Autodesk Inventor part; units mm, degrees
ref_plane "Work Plane1" through (6, 0, 0) normal (0, 0.5, 0.866) x (1, 0, 0)
ref_plane "YZ Plane" through (0, 0, 0) normal (1, 0, 0) x (0, 1, 0)
ref_plane "XZ Plane" through (0, 0, 0) normal (0, 1, 0) x (-1, 0, 0)
sketch "Sketch1" plane through (0, 0, 0) normal (0, 0, 1) x (1, 0, 0)
  line L0 (0, 0) -> (9.7226, 0)
  line L1 (12, 1.866) -> (12, 2.5)
  line L2 (12, 2.5) -> (0, 2.5)
  line L3 (12, 1.866) -> (10.8, 1.866)
  line L4 (10.8, 1.866) -> (9.7226, 0)
  line L5 (0, -0.5) -> (0, 3)
  line L6 (0, 2.5) -> (0, 0)
  dimension "d0" = 1.2
  dimension "d1" = 60
  dimension "d2" = 5
  dimension "d3" = 3.7321
  dimension "d5" = 12
revolve "Body" add sketch "Sketch1" angle 360 about axis through (0, 0, 0) along (1, 0, 0)
chamfer "Chamfer1" distance 0.3067 angle 60 1 edges at (12, -2.5, 0) measured on face at (12, 2.2645, -0.1994)
sketch "Sketch2" plane through (12, 0, 0) normal (1, 0, 0) x (0, 0, -1)
  circle A0 centre (0, 0) radius 1.866
  line L0 (-0.933, 1.616) -> (0.933, 1.616)
  line L1 (0.933, 1.616) -> (1.866, 0)
  line L2 (1.866, 0) -> (0.933, -1.616)
  line L3 (0.933, -1.616) -> (-0.933, -1.616)
  line L4 (-0.933, -1.616) -> (-1.866, 0)
  line L5 (-1.866, 0) -> (-0.933, 1.616)
  point P0 (0, 0)
  point P1 (0, 0)
extrude "Slot" add sketch "Sketch2" against normal up to next contours L1 A0 | A0 L2 | L0 A0 | A0 L3 | L5 A0 | A0 L4
thread "Thread"
chamfer "Chamfer2" distance 0.3067 angle 60 1 edges at (0, -2.5, 0) measured on face at (3.8229, 2.4919, -0.2012)
ref_plane "Work Plane1" through (6, 0, 0) normal (0, 0.5, 0.866) x (1, 0, 0)
equation "\"d0\" = INTI"
equation "\"d7\" = -0.5 * GD1 + 0.5 * NND"
equation "\"d8\" = FAWI"
equation "\"d29\" = -0.5 * GD1 + 0.5 * NND"
equation "\"d13\" = -0.5 * GD1 + 0.5 * NND"
equation "\"d14\" = FAWI"
equation "\"d30\" = -0.5 * GD1 + 0.5 * NND"
equation "\"NND\" = 3"
equation "\"NLG\" = 3"
equation "\"INTI\" = 1.2"
equation "\"FAWI\" = 60deg"
equation "\"SW\" = 1.5"
equation "\"GD1\" = THREADDIA - 1.2269 * PTC"
equation "\"FAWI1\" = 45deg"
equation "\"GUL\" = 0.61345 * PTC"
equation "\"SPD\" = 2"
equation "\"SEWI\" = 120deg"
equation "\"TOA\" = 30deg"
equation "\"THREADDIA\" = 3"
equation "\"PTC\" = 0.5"
equation "\"GAL\" = 0.61345 * PTC"
equation "\"E0\" = 1.155 * SW"
properties part number "Grub Screw 5x12mm" material "Stainless Steel, 440C"
Here's how the part is built. I have some questions about the finished solid (model axes, mm). A direction names the side the tool comes from. Coordinates: 2 decimals unless noted, no trailing zeros. Order: outer loops, then holes, each group sorted by start corner. A loop starts at its lowest first (then second) coordinate and runs counter-clockwise, first axis right, second up.
1) We'd pull the mould along Z, two halves only. Please class faces 3 (the face through (0, 0, 0)), 4 (the face through (5.81, -0.54, 2.44)), 5 (the face through (11.337, 0.819, -1.393)): +Z half, -Z half, draft (parallel to the pull), parting line (faces both ways), or undercut.
2) Will these pins go through, and if not, where does the flat tip stop? pin 1 (2 mm diameter, centred on x = 4, z = 2, fed in from +Y); pin 2 (1 mm diameter, centred on x = 9.5, y = 1.5, fed in from -Z).
3) Which directions (+Z, -Z, +X, -X, +Y, -Y) give clear straight access to the entire face, cutting with the end or side of a thin tool? Please do faces 1 (the face through (11.337, -0.797, -1.406)), 2 (the face through (12, -2, 0)).
4) I need wall thicknesses on line 1 (Y direction, x = 11, z = -0.55); line 2 (Y direction, x = 10.75, z = -0.35); line 3 (Y direction, x = 4.5, z = 1.2). Which ranges of each line are inside material? Lowest first, please.
5) Imagine slicing it at A-A on x = 1.5. List the corners of the cut face in (y, z) for me.
Response values:
1. face 3: draft
1. face 4: parting line
1. face 5: undercut
2. pin 1: stops at y = 2.29
2. pin 2: stops at z = -2.29
3. face 1: +X
3. face 2: +Z, -Z, +X, +Y, -Y
4. line 1: y = -2.44 to -1.62, 1.62 to 2.44
4. line 2: y = -2.48 to -1.62, 1.62 to 2.48
4. line 3: y = -2.19 to 2.19
5. outline: circle Ø5 at (0, 0)
